Verification items for the finished model (mm, model axes). Face numbers are marked on the shaded views. A direction names the side the tool comes from. Give positions to 0.01 mm unless a question says otherwise; leave off trailing zeros. Order: outer loops, then holes, each group sorted by start corner. A loop starts at its lowest first (then second) coordinate and runs counter-clockwise, first axis right, second up. Notation, with made-up numbers: (59, -20.5) - (94, -20.5) arc R17 ccw to (94, -4.5) - close; hole circle Ø4 at (33.5, 68.5). An arc over 180 degrees is marked (long way). Answer as a JSON object with one key per item and string values. Group by question number.
(1) Mould release check, pull along X, two halves, no side actions. Record for the marked faces 3, 4, 5 and 6: +X half, -X half, draft (parallel to the pull), parting line (faces both ways), or undercut.
(2) Section check A-A (y = 9.75). Record the boundary of the cut face in (x, z) (3 decimals), then the cut area to 3 significant figures.
(3) Access from +Z, -Z, +X, -X, +Y, -Y to the whole of each face (thin tool, end or side, straight path). Record for the marked faces 1 and 2.
(4) Section check D-D (y = 7.75). Record the boundary of the cut face in (x, z).
(5) Thickness scan on line 1 (Z direction, x = -1.25, y = 9.25); line 2 (Z direction, x = 0, y = 7.75); line 3 (Y direction, x = -0.5, z = -11). Record the ranges inside material, lowest first.
(6) Section check C-C (x = 0). Count the separate pieces of the cut face and the enclosed holes in it, then the cut area to 3 significant figures.
(7) Section check B-B (z = 0). Record the boundary of the cut face in (x, y).
(8) Depth check by flat-ended pin: pin 1 Ø2.5 at (x, z) = (0, -14.605) entering from +Y; pin 2 Ø4 at (y, z) = (3.5, 7.5) entering from +X; pin 3 Ø1.5 at (x, y) = (-8, 5) entering from +Z; pin 4 Ø1.5 at (x, y) = (-0.5, 7.5) entering from +Z. Enter the tip coordinate at first touch or a pass-through.
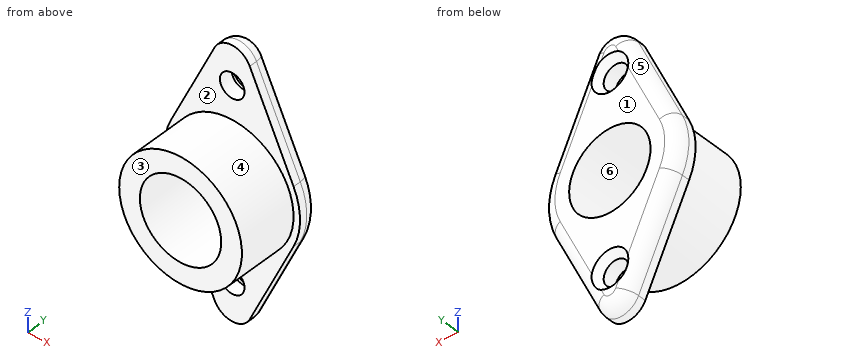
Autodesk Inventor part; units mm, degrees
ref_plane "YZ Plane" through (0, 0, 0) normal (1, 0, 0) x (0, 1, 0)
ref_plane "XZ Plane" through (0, 0, 0) normal (0, 1, 0) x (-1, 0, 0)
ref_plane "XY Plane" through (0, 0, 0) normal (0, 0, 1) x (1, 0, 0)
sketch "Sketch1" plane through (0, 0, 0) normal (0, 1, 0) x (-1, 0, 0)
  circle A0 centre (0, 0) radius 9.5
  dimension "Cutout_Diameter" = 19
extrude "Extrusion1" add sketch "Sketch1" along normal blind 9.2
sketch "Sketch2" plane through (0, 9.2, 0) normal (0, 1, 0) x (1, 0, 0)
  line L0 (0, 0) -> (0, 17.625) construction
  line L1 (0, 0) -> (0, -17.625) construction
  arc A0 (-2.7148, -18.9016) -> (2.7148, -18.9016) centre (0, -17.625) ccw
  arc A1 (2.7148, 18.9016) -> (-2.7148, 18.9016) centre (0, 17.625) ccw
  line L2 (-2.7148, -18.9016) -> (-9.5019, -4.4681)
  line L3 (-9.5019, 4.4681) -> (-2.7148, 18.9016)
  line L4 (2.7148, 18.9016) -> (9.5019, 4.4681)
  line L5 (9.5019, -4.4681) -> (2.7148, -18.9016)
  arc A2 (9.5019, -4.4681) -> (9.5019, 4.4681) centre (0, 0) ccw
  arc A3 (-9.5019, 4.4681) -> (-9.5019, -4.4681) centre (0, 0) ccw
  dimension "Mount_Tip_Radius" = 6
  dimension "Mount_Center_Radius" = 10.5
  dimension "Mount_Tip_Length" = 41.25
extrude "Extrusion2" add sketch "Sketch2" along normal blind 3.2
sketch "Sketch3" plane through (0, 12.4, 0) normal (0, 1, 0) x (1, 0, 0)
  line L0 (0, -14.605) -> (0, 14.605) construction
  point P0 (0, 0)
  point P1 (0, 0)
  dimension "Mount_Hole_Spacing" = 29.21
hole "Hole1" at (0, 12.4, 14.605) at (0, 12.4, -14.605) direction (0, -1, 0) diameter 3.81 end through all countersink diameter 5.715 countersink angle 82
sketch "Sketch4" plane through (0, 12.4, 0) normal (0, 1, 0) x (1, 0, 0)
  point P0 (0, 0)
  point P1 (0, 0)
hole "Hole2" at (0, 12.4, 0) direction (0, -1, 0) diameter 12.6 end through all
fillet "Fillet1" radius 2 8 edges at (10.5, 12.4, 0) (6.1084, 12.4, -11.6848) (0, 12.4, -20.625) (-6.1084, 12.4, -11.6848) (-10.5, 12.4, 0) (-6.1084, 12.4, 11.6848) (0, 12.4, 20.625) (6.1084, 12.4, 11.6848)
properties part number "Deck_Bushing_Outer" material "Nylon 6/6"
Solutions:
{
 "1": {"face 3": "draft", "face 4": "parting line", "face 5": "-X half", "face 6": "undercut"},
 "2": {"outline": "(-9.502, -4.468) - (-2.715, -18.902) arc R3 ccw to (2.715, -18.902) - (9.502, -4.468) arc R10.5 ccw to (9.502, 4.468) - (2.715, 18.902) arc R3 ccw to (-2.715, 18.902) - (-9.502, 4.468) arc R10.5 ccw to start; hole circle Ø12.6 at (0, 0); hole circle Ø3.81 at (0, -14.605); hole circle Ø3.81 at (0, 14.605)", "area": "400 mm2"},
 "3": {"face 1": "+Z, -Z, +X, -X, +Y", "face 2": "-Y"},
 "4": {"outline": "circle Ø19 at (0, 0); hole circle Ø12.6 at (0, 0)"},
 "5": {"line 1": "z = -20.35 to -16.04, -13.17 to -6.17, 6.17 to 13.17, 16.04 to 20.35", "line 2": "z = -9.5 to -6.3, 6.3 to 9.5", "line 3": "y = 9.2 to 12.4"},
 "6": {"separate pieces": "4", "enclosed holes": "0", "area": "122 mm2"},
 "7": {"outline": "(-10.5, 9.2) - (-9.5, 9.2) - (-9.5, 0) - (-6.3, 0) - (-6.3, 12.4) - (-8.5, 12.4) arc R2 ccw to (-10.5, 10.4) - close; (6.3, 0) - (9.5, 0) - (9.5, 9.2) - (10.5, 9.2) - (10.5, 10.4) arc R2 ccw to (8.5, 12.4) - (6.3, 12.4) - close"},
 "8": {"pin 1": "passes through", "pin 2": "stops at x = 7.75", "pin 3": "stops at z = 6.14", "pin 4": "stops at z = 9.5"}
}
